Verification items for this drawing (mm, ordinates from the low corner). Round coordinates to 2 decimals unless told otherwise and drop trailing zeros. Order: outer loops, then holes, each group sorted by start corner. A loop starts at its lowest first (then second) coordinate and runs counter-clockwise, first axis right, second up.
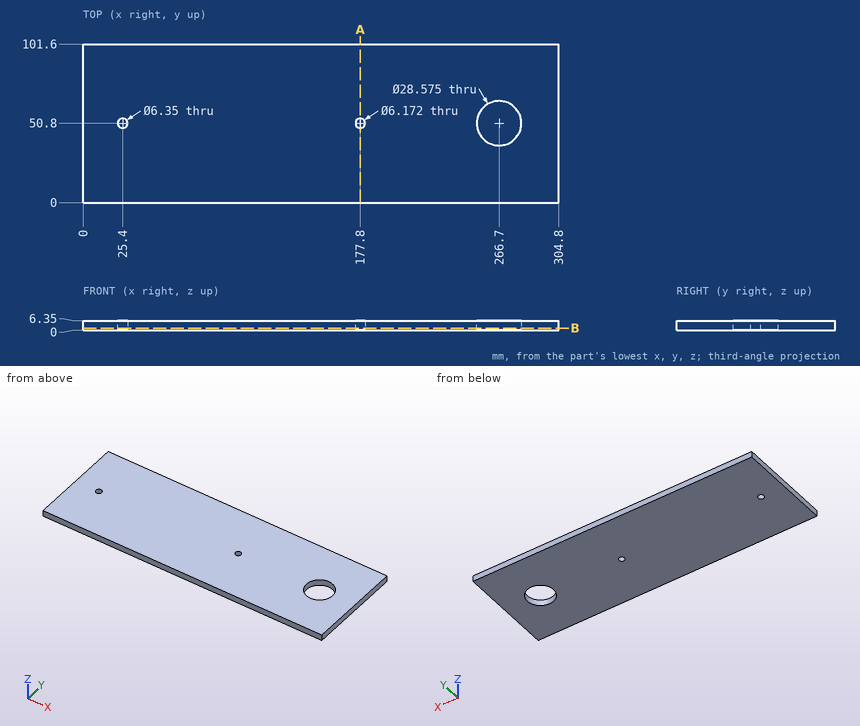
Item 1: Sectioned sample at A-A (x = 177.8). Record the cut outline in (y, z), and give its area (3 significant figures).
Answer:
outline: (0, 0) - (47.71, 0) - (47.71, 6.35) - (0, 6.35) - close; (53.89, 0) - (101.6, 0) - (101.6, 6.35) - (53.89, 6.35) - close
area: 606 mm2
Item 2: Scan lines: line 1 along Y through (x, z) = (177.8, 2.5); line 2 along Y through (x, z) = (25.4, 4.75) (3 decimals); line 3 along X through (y, z) = (53, 3.5) (1 decimal). Record each from-to range of solid material in increasing order.
Answer:
line 1: y = 0 to 47.71, 53.89 to 101.6
line 2: y = 0 to 47.625, 53.975 to 101.6
line 3: x = 0 to 23.1, 27.7 to 175.6, 180 to 252.6, 280.8 to 304.8
Item 3: Sectioned sample at B-B (z = 1.5). State how many separate pieces and enclosed holes the cut face has, and give its area (3 significant figures).
Answer:
separate pieces: 1
enclosed holes: 3
area: 30,300 mm2
Item 4: Go/stop test with flat-tipped pins: P1, Ø3.5, axis at x = 177.8, y = 50.8, coming from the -Z side; P2, Ø1, axis at x = 47.5, z = 2, coming from the -Y side. Record where each tip stops, or that it passes through.
Answer:
P1: passes through
P2: stops at y = 0
